```python
from build123d import *

# Parameters (mm, degrees)
SKETCH1_W                   = 200
SKETCH1_H                   = 100
BOSS_EXTRUDE1_DEPTH         = 25
SKETCH2_R                   = 6.35
CUT_EXTRUDE1_DEPTH          = 87.5
SKETCH3_R                   = 6.35
CUT_EXTRUDE2_DEPTH          = 19
CUT_EXTRUDE3_REACH          = 27
SKETCH4_R                   = 6.35
CUT_EXTRUDE4_DEPTH          = 6.35
F_1_4_20_TAPPED_HOLE1_D     = 5.1054
F_1_4_20_TAPPED_HOLE1_DEPTH = 25


with BuildPart() as part:
    # Sketch1 → Boss-Extrude1 (new body)
    with BuildSketch(Plane(origin=(0, 0, 0), x_dir=(1, 0, 0), z_dir=(0, 1, 0))):
        Rectangle(SKETCH1_W, SKETCH1_H)
    extrude(amount=BOSS_EXTRUDE1_DEPTH)

    # Sketch2 → Cut-Extrude1 (cut)
    with BuildSketch(Plane.XY.offset(50)):
        with Locations((-75, 12.5)):
            Circle(SKETCH2_R)
        with Locations((87.500000108, 12.5)):
            Circle(SKETCH2_R)
    extrude(amount=-CUT_EXTRUDE1_DEPTH, mode=Mode.SUBTRACT)

    # Sketch3 → Cut-Extrude2 (cut)
    with BuildSketch(Plane(origin=(0, 25, 0), x_dir=(1, 0, 0), z_dir=(0, 1, 0))):
        with Locations((-75, 12.5)):
            Circle(SKETCH3_R)
        with Locations((-75, -25)):
            Circle(SKETCH3_R)
        with Locations((87.500000108, -6.25)):
            Circle(SKETCH3_R)
    extrude(amount=-CUT_EXTRUDE2_DEPTH, mode=Mode.SUBTRACT)

    # Sketch4 → Cut-Extrude3 (cut, up to next)
    with BuildSketch(Plane(origin=(0, 25, 0), x_dir=(1, 0, 0), z_dir=(0, 1, 0)), mode=Mode.PRIVATE) as cut_extrude3_sk1:
        with Locations((6.25, -6.25)):
            Circle(SKETCH4_R)
    cut_extrude3_tool1 = extrude(cut_extrude3_sk1.sketch, amount=-CUT_EXTRUDE3_REACH, mode=Mode.PRIVATE) & part.part
    add(cut_extrude3_tool1.solids().sort_by_distance((6.25, 25, 6.25))[0], mode=Mode.SUBTRACT)

    # Sketch5 → Cut-Extrude4 (cut)
    with BuildSketch(Plane(origin=(0, 0, 0), x_dir=(-1, 0, 0), z_dir=(0, -1, 0))):
        with BuildLine():
            Line((-9.425, 7.143897512), (-9.425, -0.750738686))
            ThreePointArc((-9.425, -0.750738686), (-6.25, 0.1), (-3.075, -0.750738686))
            Line((-3.075, -0.750738686), (-3.075, 7.143897512))
            ThreePointArc((-3.075, 7.143897512), (-6.25, 10.318897512), (-9.425, 7.143897512))
        make_face()
        with BuildLine():
            Line((-9.425, -11.749261314), (-9.425, -18.256102488))
            ThreePointArc((-9.425, -18.256102488), (-6.25, -21.431102488), (-3.075, -18.256102488))
            Line((-3.075, -18.256102488), (-3.075, -11.749261314))
            ThreePointArc((-3.075, -11.749261314), (-6.25, -12.6), (-9.425, -11.749261314))
        make_face()
    extrude(amount=-CUT_EXTRUDE4_DEPTH, mode=Mode.SUBTRACT)

    # 1/4-20 Tapped Hole1
    with Locations(Plane(origin=(-75, 25, -43.75), x_dir=(0, 0, 1), z_dir=(0, 1, 0))):
        with Locations((0, 0), (0, 150), (18.75, -18.75), (68.75, -18.75)):
            Hole(F_1_4_20_TAPPED_HOLE1_D / 2, depth=F_1_4_20_TAPPED_HOLE1_DEPTH)


solid = part.part
```
Verification items for the finished model (mm, model axes). A direction names the side the tool comes from. Give positions to 0.01 mm unless a question says otherwise; leave off trailing zeros. Order: outer loops, then holes, each group sorted by start corner. A loop starts at its lowest first (then second) coordinate and runs counter-clockwise, first axis right, second up. Notation, with made-up numbers: M 78.25,9.25 L 135.25,9.25 A20 ccw 135.25,16.25 Z; hole C -34,-25 d9. An arc over 180 degrees is marked long. Answer in a Markdown table with one row per item. Add a question column.
Item 1: Section check D-D, the plane x = -93.75. Enter the section's corners in (y, z).
Item 2: Scan lines: probe 1 along X at (y, z) = (12.5, 31.25); probe 2 along X at (y, z) = (12.5, 23.5); probe 3 along X at (y, z) = (8.5, -12.5). Record each from-to range of solid material in increasing order. Write a range as from..to.
Item 3: Gauge pin test, flat ends, axial feed: pin 1 (11.5 mm diameter, centred on x = 87.5, y = 12.5, fed in from +Z); pin 2 (3 mm diameter, centred on x = 7.5, z = -3.5, fed in from -Y); pin 3 (10 mm diameter, centred on x = -75, z = -12.5, fed in from +Y). Record the tip position at first contact, or that the pin passes through.
Item 4: Mould release check, pull along Z, two halves, no side actions. Record for faces 1 (the flat face through (-1, 12, 50)), 2 (the flat face through (87, 6, 6)), 3 (the flat face through (100, 12, 1)), 4 (the flat face through (-1, 12, -50)): released by +Z, released by -Z, zero draft, split by the parting line, or undercut.
Item 5: Section check A-A, the plane x = 87.5. Enter the section's corners in (y, z).
Item 6: Section check B-B, the plane z = -25. Enter the section's corners in (x, y), and give its area (3 significant figures).
Item 7: Tool access check on faces 5 (the flat face through (-1, 0, -1)), 6 (the cylindrical face through (93.366, 10.068, 28.431)), 7 (the cylindrical face through (6.18, 3.13, -10.32)), 8 (the cylindrical face through (82.82, 20.23, 1.96)). Record the directions out of +Z, -Z, +X, -X, +Y, -Y that give a thin tool (end or side, any length) a straight path to the whole face; none if there is none.
Item 8: Section check C-C, the plane y = 3.5. Enter the section's corners in (x, z) (3 decimals).
Filled sheet:
| question | item | result |
|---|---|---|
| 1 | outline | M 0,-50 L 25,-50 L 25,-27.55 L 0,-27.55 Z; M 0,-22.45 L 25,-22.45 L 25,22.45 L 0,22.45 Z; M 0,27.55 L 25,27.55 L 25,50 L 0,50 Z |
| 2 | probe 1 | x = -100..-81.35, -68.65..81.15, 93.85..100 |
| 2 | probe 2 | x = -100..-95.82, -91.68..-81.35, -68.65..81.15, 93.85..100 |
| 2 | probe 3 | x = -100..-81.35, -68.65..82.57, 92.43..100 |
| 3 | pin 1 | stops at z = -37.5 |
| 3 | pin 2 | stops at y = 6.35 |
| 3 | pin 3 | stops at y = 6 |
| 4 | face 1 | released by +Z |
| 4 | face 2 | undercut |
| 4 | face 3 | zero draft |
| 4 | face 4 | released by -Z |
| 5 | outline | M 0,-50 L 25,-50 L 25,-0.1 L 18.85,-0.1 L 18.85,-37.5 L 6.15,-37.5 L 6.15,-0.1 L 6,-0.1 L 6,12.6 L 6.15,12.6 L 6.15,50 L 0,50 Z; M 18.85,12.6 L 25,12.6 L 25,50 L 18.85,50 Z |
| 6 | outline | M -100,0 L -96.3,0 L -96.3,25 L -100,25 Z; M -91.2,0 L 100,0 L 100,25 L -91.2,25 Z; hole C -75,12.5 d12.7; hole C 87.5,12.5 d12.7 |
| 6 | area | 4,620 mm^2 |
| 7 | face 5 | +Z, -Z, +X, -X, -Y |
| 7 | face 6 | +Z |
| 7 | face 7 | -Y |
| 7 | face 8 | +Y |
| 8 | outline | M -100,-50 L 100,-50 L 100,50 L -100,50 Z; hole C -93.75,-25 d5.105; hole C -93.75,25 d5.105; hole C -75,-43.75 d5.105; hole M 3.075,-7.144 A3.175 ccw 9.425,-7.144 L 9.425,0.751 A6.35 ccw 9.425,11.749 L 9.425,18.256 A3.175 ccw 3.075,18.256 L 3.075,11.749 A6.35 ccw 3.075,0.751 Z; hole C 75,-43.75 d5.105 |
